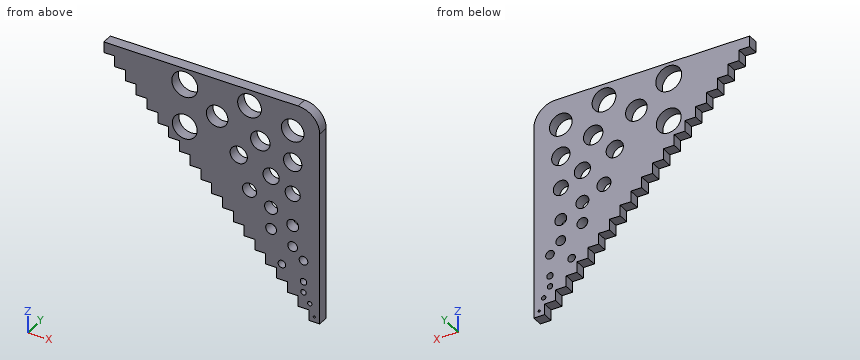
from build123d import *

# Parameters (mm, degrees)
BOSS_EXTRUDE1_OUTLINE_R    = 6
BOSS_EXTRUDE1_OUTLINE_R_2  = 5.75
BOSS_EXTRUDE1_OUTLINE_R_3  = 5.5
BOSS_EXTRUDE1_OUTLINE_R_4  = 5
BOSS_EXTRUDE1_OUTLINE_R_5  = 4.5
BOSS_EXTRUDE1_OUTLINE_R_6  = 5.25
BOSS_EXTRUDE1_OUTLINE_R_7  = 4
BOSS_EXTRUDE1_OUTLINE_R_8  = 3.25
BOSS_EXTRUDE1_OUTLINE_R_9  = 4.25
BOSS_EXTRUDE1_OUTLINE_R_10 = 3.75
BOSS_EXTRUDE1_OUTLINE_R_11 = 3.5
BOSS_EXTRUDE1_OUTLINE_R_12 = 3
BOSS_EXTRUDE1_OUTLINE_R_13 = 2.75
BOSS_EXTRUDE1_OUTLINE_R_14 = 2.5
BOSS_EXTRUDE1_OUTLINE_R_15 = 2.25
BOSS_EXTRUDE1_OUTLINE_R_16 = 2
BOSS_EXTRUDE1_OUTLINE_R_17 = 1.75
BOSS_EXTRUDE1_OUTLINE_R_18 = 1.5
BOSS_EXTRUDE1_OUTLINE_R_19 = 1.25
BOSS_EXTRUDE1_OUTLINE_R_20 = 1
BOSS_EXTRUDE1_OUTLINE_R_21 = 0.5
BOSS_EXTRUDE1_DEPTH        = 5
FILLET1_R                  = 10


# Read off the part's stored shape, not the designer's step: Boss-Extrude1
with BuildPart() as part:
    # Boss-Extrude1 outline → Boss-Extrude1 (new body)
    with BuildSketch(Plane(origin=(0, 0, 0), x_dir=(1, 0, 0), z_dir=(0, 1, 0))):
        Polygon((60, 65), (60, 60), (55, 60), (55, 55), (50, 55), (50, 50), (45, 50), (45, 45), (40, 45), (40, 40), (35, 40), (35, 35), (30, 35), (30, 30), (25, 30), (25, 25), (20, 25), (20, 20), (15, 20), (15, 15), (10, 15), (10, 10), (5, 10), (5, 5), (0, 5), (0, 0), (100, 0), (100, 100), (95, 100), (95, 95), (90, 95), (90, 90), (85, 90), (85, 85), (80, 85), (80, 80), (75, 80), (75, 75), (70, 75), (70, 70), (65, 70), (65, 65), align=None)
        with Locations((37.5, 7.5)):
            Circle(BOSS_EXTRUDE1_OUTLINE_R, mode=Mode.SUBTRACT)
        with Locations((37.5, 27.5)):
            Circle(BOSS_EXTRUDE1_OUTLINE_R_2, mode=Mode.SUBTRACT)
        with Locations((67.5, 7.5)):
            Circle(BOSS_EXTRUDE1_OUTLINE_R_3, mode=Mode.SUBTRACT)
        with Locations((52.5, 17.5)):
            Circle(BOSS_EXTRUDE1_OUTLINE_R_4, mode=Mode.SUBTRACT)
        with Locations((72.5, 22.5)):
            Circle(BOSS_EXTRUDE1_OUTLINE_R_5, mode=Mode.SUBTRACT)
        with Locations((87.5, 12.5)):
            Circle(BOSS_EXTRUDE1_OUTLINE_R_6, mode=Mode.SUBTRACT)
        with Locations((62.5, 32.5)):
            Circle(BOSS_EXTRUDE1_OUTLINE_R_7, mode=Mode.SUBTRACT)
        with Locations((67.5, 47.5)):
            Circle(BOSS_EXTRUDE1_OUTLINE_R_8, mode=Mode.SUBTRACT)
        with Locations((87.5, 27.5)):
            Circle(BOSS_EXTRUDE1_OUTLINE_R_9, mode=Mode.SUBTRACT)
        with Locations((77.5, 37.5)):
            Circle(BOSS_EXTRUDE1_OUTLINE_R_10, mode=Mode.SUBTRACT)
        with Locations((87.5, 42.5)):
            Circle(BOSS_EXTRUDE1_OUTLINE_R_11, mode=Mode.SUBTRACT)
        with Locations((77.5, 52.5)):
            Circle(BOSS_EXTRUDE1_OUTLINE_R_12, mode=Mode.SUBTRACT)
        with Locations((87.5, 57.5)):
            Circle(BOSS_EXTRUDE1_OUTLINE_R_13, mode=Mode.SUBTRACT)
        with Locations((77.5, 62.5)):
            Circle(BOSS_EXTRUDE1_OUTLINE_R_14, mode=Mode.SUBTRACT)
        with Locations((87.5, 67.5)):
            Circle(BOSS_EXTRUDE1_OUTLINE_R_15, mode=Mode.SUBTRACT)
        with Locations((92.5, 72.5)):
            Circle(BOSS_EXTRUDE1_OUTLINE_R_16, mode=Mode.SUBTRACT)
        with Locations((82.5, 77.5)):
            Circle(BOSS_EXTRUDE1_OUTLINE_R_17, mode=Mode.SUBTRACT)
        with Locations((92.5, 82.5)):
            Circle(BOSS_EXTRUDE1_OUTLINE_R_18, mode=Mode.SUBTRACT)
        with Locations((92.5, 87.5)):
            Circle(BOSS_EXTRUDE1_OUTLINE_R_19, mode=Mode.SUBTRACT)
        with Locations((95.397156107, 91.933376666)):
            Circle(BOSS_EXTRUDE1_OUTLINE_R_20, mode=Mode.SUBTRACT)
        with Locations((97.5, 97.5)):
            Circle(BOSS_EXTRUDE1_OUTLINE_R_21, mode=Mode.SUBTRACT)
    extrude(amount=BOSS_EXTRUDE1_DEPTH)

    # Fillet1
    fillet1_edges = [part.edges().sort_by_distance(p)[0] for p in [
        (100, 2.5, 0),
    ]]
    fillet(fillet1_edges, radius=FILLET1_R)


solid = part.part
Work out the finished part from the listing and answer in its coordinate system (mm). Give positions to 0.01 mm unless a question says otherwise; leave off trailing zeros. Order: outer loops, then holes, each group sorted by start corner. A loop starts at its lowest first (then second) coordinate and runs counter-clockwise, first axis right, second up. Notation, with made-up numbers: (-29, 28) -> (24, 28) arc R23 cw to (24, 43) -> close; hole circle Ø6 at (64, 8). An arc over 180 degrees is marked (long way). Answer as a JSON object with one key per item and string values. Group by question number.
1. Section C-C on x = 87.5 is taken. Determine the outline of the cut face in (y, z).
2. Section B-B on z = -47.5 is taken. Determine the outline of the cut face in (x, y), plus the area to 4 significant figures.
3. Section D-D on x = 52.5 is taken. Determine the outline of the cut face in (y, z).
4. Section A-A on x = 37.5 is taken. Determine the outline of the cut face in (y, z), plus the area to 3 significant figures.
5. Flat-ended cylindrical pins translate along their axes: pin 1 Ø2.5 at (y, z) = (3.5, -72) entering from -X; pin 2 Ø1.5 at (x, y) = (46.5, 3.5) entering from -Z; pin 3 Ø2.5 at (x, y) = (51.5, 2) entering from -Z; pin 4 Ø9 at (x, z) = (52.5, -17.5) entering from -Y. Find the tip coordinate at first contact, or state that the pin passes through.
6. Consider line 1 along Z through (x, y) = (37.5, 1.05); line 2 along Z through (x, y) = (77.5, 2.15); line 3 along X through (y, z) = (2.1, -87.5). Determine where each line is inside the solid, lowest interval first. Write a range as [from, to].
Result sheet:
{
 "1": {"outline": "(0, -90) -> (5, -90) -> (5, -69.75) -> (0, -69.75) -> close; (0, -65.25) -> (5, -65.25) -> (5, -60.25) -> (0, -60.25) -> close; (0, -54.75) -> (5, -54.75) -> (5, -46) -> (0, -46) -> close; (0, -39) -> (5, -39) -> (5, -31.75) -> (0, -31.75) -> close; (0, -23.25) -> (5, -23.25) -> (5, -17.75) -> (0, -17.75) -> close; (0, -7.25) -> (5, -7.25) -> (5, 0) -> (0, 0) -> close"},
 "2": {"outline": "(45, 0) -> (64.25, 0) -> (64.25, 5) -> (45, 5) -> close; (70.75, 0) -> (100, 0) -> (100, 5) -> (70.75, 5) -> close", "area": "242.5 mm^2"},
 "3": {"outline": "(0, -55) -> (5, -55) -> (5, -22.5) -> (0, -22.5) -> close; (0, -12.5) -> (5, -12.5) -> (5, 0) -> (0, 0) -> close"},
 "4": {"outline": "(0, -40) -> (5, -40) -> (5, -33.25) -> (0, -33.25) -> close; (0, -21.75) -> (5, -21.75) -> (5, -13.5) -> (0, -13.5) -> close; (0, -1.5) -> (5, -1.5) -> (5, 0) -> (0, 0) -> close", "area": "82.5 mm^2"},
 "5": {"pin 1": "stops at x = 70", "pin 2": "stops at z = -50", "pin 3": "stops at z = -55", "pin 4": "passes through"},
 "6": {"line 1": "z = [-40, -33.25], [-21.75, -13.5], [-1.5, 0]", "line 2": "z = [-80, -65], [-60, -55.5], [-49.5, -41.25], [-33.75, 0]", "line 3": "x = [85, 91.25], [93.75, 100]"}
}
